Source: CAD feature listing. Evaluate the final solid. Frame: model axes, mm. A direction names the side the tool comes from. Round coordinates to 2 decimals unless told otherwise and drop trailing zeros. Write each loop counter-clockwise with the first axis right and the second up, starting at its lowest first coordinate (ties: lowest second). Pieces come first, ordered by that corner, then holes. Notation, with made-up numbers: (86, -24.5) - (95, -24.5) arc R16 ccw to (95, -16.5) - close; hole circle Ø2 at (89.25, 7). An arc over 180 degrees is marked (long way). Write item = value, one per line. Start each with the question number.
```python
from build123d import *

# Parameters (mm, degrees)
SKETCH1_W      = 16
SKETCH1_H      = 16
EXTRUDE1_DEPTH = 112
SKETCH2_W      = 13
SKETCH2_H      = 13
EXTRUDE2_DEPTH = 115.262854857
SKETCH3_R      = 4
SKETCH3_R_2    = 1.85
EXTRUDE3_DEPTH = 115.262854857
SKETCH4_R      = 4
SKETCH4_R_2    = 1.85
EXTRUDE4_DEPTH = 115.262854857
FILLET1_R      = 1


with BuildPart() as part:
    # Sketch1 → Extrude1 (new body)
    with BuildSketch(Plane.XY):
        with Locations((8, 8)):
            Rectangle(SKETCH1_W, SKETCH1_H)
    extrude(amount=-EXTRUDE1_DEPTH)

    # Sketch2 → Extrude2 (cut, through all)
    with BuildSketch(Plane.XY):
        with Locations((8, 8)):
            Rectangle(SKETCH2_W, SKETCH2_H)
    extrude(amount=-EXTRUDE2_DEPTH, mode=Mode.SUBTRACT)

    # Sketch3 → Extrude3 (cut, through all)
    with BuildSketch(Plane(origin=(0, 16, 0), x_dir=(1, 0, 0), z_dir=(0, 1, 0))):
        with Locations(Location((8, 64, 0), (0, 0, 270))):
            Circle(SKETCH3_R)
        with Locations(Location((8, 32, 0), (0, 0, 270))):
            Circle(SKETCH3_R)
        with Locations((8, 0)):
            Circle(SKETCH3_R)
        with Locations(Location((8, 96, 0), (0, 0, 270))):
            Circle(SKETCH3_R)
        with Locations((8, 128)):
            Circle(SKETCH3_R)
        with Locations((8, 160)):
            Circle(SKETCH3_R)
        with Locations((8, 192)):
            Circle(SKETCH3_R)
        with Locations((8, 224)):
            Circle(SKETCH3_R)
        with Locations((8, 256)):
            Circle(SKETCH3_R)
        with Locations(Location((8, 48, 0), (0, 0, 270))):
            Circle(SKETCH3_R)
        with Locations(Location((8, 56, 0), (0, 0, 270))):
            Circle(SKETCH3_R_2)
        with Locations(Location((8, 40, 0), (0, 0, 270))):
            Circle(SKETCH3_R_2)
        with Locations(Location((8, 80, 0), (0, 0, 270))):
            Circle(SKETCH3_R)
        with Locations(Location((8, 88, 0), (0, 0, 270))):
            Circle(SKETCH3_R_2)
        with Locations(Location((8, 72, 0), (0, 0, 270))):
            Circle(SKETCH3_R_2)
        with Locations(Location((8, 16, 0), (0, 0, 270))):
            Circle(SKETCH3_R)
        with Locations(Location((8, 24, 0), (0, 0, 270))):
            Circle(SKETCH3_R_2)
        with Locations(Location((8, 8, 0), (0, 0, 270))):
            Circle(SKETCH3_R_2)
        with Locations((8, 112)):
            Circle(SKETCH3_R)
        with Locations((8, 120)):
            Circle(SKETCH3_R_2)
        with Locations(Location((8, 104, 0), (0, 0, 270))):
            Circle(SKETCH3_R_2)
        with Locations((8, 144)):
            Circle(SKETCH3_R)
        with Locations((8, 152)):
            Circle(SKETCH3_R_2)
        with Locations((8, 136)):
            Circle(SKETCH3_R_2)
        with Locations((8, 176)):
            Circle(SKETCH3_R)
        with Locations((8, 184)):
            Circle(SKETCH3_R_2)
        with Locations((8, 168)):
            Circle(SKETCH3_R_2)
        with Locations((8, 208)):
            Circle(SKETCH3_R)
        with Locations((8, 216)):
            Circle(SKETCH3_R_2)
        with Locations((8, 200)):
            Circle(SKETCH3_R_2)
        with Locations((8, 240)):
            Circle(SKETCH3_R)
        with Locations((8, 248)):
            Circle(SKETCH3_R_2)
        with Locations((8, 232)):
            Circle(SKETCH3_R_2)
    extrude(amount=-EXTRUDE3_DEPTH, mode=Mode.SUBTRACT)

    # Sketch4 → Extrude4 (cut, through all)
    with BuildSketch(Plane(origin=(16, 0, 0), x_dir=(0, 0, -1), z_dir=(1, 0, 0))):
        with Locations(Location((32, 8, 0), (0, 0, 90))):
            Circle(SKETCH4_R)
        with Locations(Location((64, 8, 0), (0, 0, 90))):
            Circle(SKETCH4_R)
        with Locations((0, 8)):
            Circle(SKETCH4_R)
        with Locations(Location((96, 8, 0), (0, 0, 90))):
            Circle(SKETCH4_R)
        with Locations((128, 8)):
            Circle(SKETCH4_R)
        with Locations((160, 8)):
            Circle(SKETCH4_R)
        with Locations((192, 8)):
            Circle(SKETCH4_R)
        with Locations((224, 8)):
            Circle(SKETCH4_R)
        with Locations((256, 8)):
            Circle(SKETCH4_R)
        with Locations(Location((48, 8.074203, 0), (0, 0, 90))):
            Circle(SKETCH4_R)
        with Locations(Location((40, 8.074203, 0), (0, 0, 90))):
            Circle(SKETCH4_R_2)
        with Locations(Location((56, 8.074203, 0), (0, 0, 90))):
            Circle(SKETCH4_R_2)
        with Locations(Location((80, 8, 0), (0, 0, 90))):
            Circle(SKETCH4_R)
        with Locations(Location((72, 8, 0), (0, 0, 90))):
            Circle(SKETCH4_R_2)
        with Locations(Location((88, 8, 0), (0, 0, 90))):
            Circle(SKETCH4_R_2)
        with Locations(Location((16, 8, 0), (0, 0, 90))):
            Circle(SKETCH4_R)
        with Locations(Location((8, 8, 0), (0, 0, 90))):
            Circle(SKETCH4_R_2)
        with Locations(Location((24, 8, 0), (0, 0, 90))):
            Circle(SKETCH4_R_2)
        with Locations((112, 8)):
            Circle(SKETCH4_R)
        with Locations(Location((104, 8, 0), (0, 0, 90))):
            Circle(SKETCH4_R_2)
        with Locations((120, 8)):
            Circle(SKETCH4_R_2)
        with Locations((144, 8)):
            Circle(SKETCH4_R)
        with Locations((136, 8)):
            Circle(SKETCH4_R_2)
        with Locations((152, 8)):
            Circle(SKETCH4_R_2)
        with Locations((176, 8)):
            Circle(SKETCH4_R)
        with Locations((168, 8)):
            Circle(SKETCH4_R_2)
        with Locations((184, 8)):
            Circle(SKETCH4_R_2)
        with Locations((208, 8)):
            Circle(SKETCH4_R)
        with Locations((200, 8)):
            Circle(SKETCH4_R_2)
        with Locations((216, 8)):
            Circle(SKETCH4_R_2)
        with Locations((240, 8)):
            Circle(SKETCH4_R)
        with Locations((232, 8)):
            Circle(SKETCH4_R_2)
        with Locations((248, 8)):
            Circle(SKETCH4_R_2)
    extrude(amount=-EXTRUDE4_DEPTH, mode=Mode.SUBTRACT)

    # Fillet1
    fillet1_edges = [part.edges().sort_by_distance(p)[0] for p in [
        (0, 16, -56),
        (16, 16, -56),
        (16, 0, -56),
        (0, 0, -56),
    ]]
    fillet(fillet1_edges, radius=FILLET1_R)


solid = part.part
```
(1) Section D-D (y = 8.5). Count the separate pieces of the cut face and the enclosed holes in it, plus the area to 3 significant figures.
(2) Contact query for a flat-ended pin moving along its axis: P1, Ø4, axis at x = 13, y = 12, coming from the +Z side. Output: stop coordinate, or through.
(3) Section A-A (z = -48). Return the cut outline in (x, y), plus the area to 3 significant figures.
(4) Reachability of faces 1 (the flat face through (0, 6, -55)), 2 (the flat face through (5, 14.5, -55)) from +Z, -Z, +X, -X, +Y, -Y: full face, straight path, thin tool, end or side. Return the list, or none.
(5) Pull-direction query (Y, two-part tool) for faces 3 (the cylindrical face through (7.29, 15.26, -102.29)), 4 (the cylindrical face through (15.26, 7.479, -28.034)); classes: +Y half, -Y half, draft (parallel to the pull), parting line (faces both ways), or undercut.
(6) Ray query, L1, parallel to X at y = 3, z = -66.5; L2, parallel to X at y = 15, z = -35. Return the intervals inside material, ascending. Write a range as from..to.
(7) Section B-B (x = 3). Return the cut outline in (y, z), plus the area to 3 significant figures.
Solution:
q1.separate_pieces = 28
q1.enclosed_holes = 0
q1.area = 94.2 mm^2
q2.P1 = 0
q3.outline = (0, 1) arc R1 ccw to (1, 0) - (4, 0) - (4, 1.5) - (1.5, 1.5) - (1.5, 4.07) - (0, 4.07) - close; (0, 12.07) - (1.5, 12.07) - (1.5, 14.5) - (4, 14.5) - (4, 16) - (1, 16) arc R1 ccw to (0, 15) - close; (12, 0) - (15, 0) arc R1 ccw to (16, 1) - (16, 4.07) - (14.5, 4.07) - (14.5, 1.5) - (12, 1.5) - close; (12, 14.5) - (14.5, 14.5) - (14.5, 12.07) - (16, 12.07) - (16, 15) arc R1 ccw to (15, 16) - (12, 16) - close
q3.area = 38.1 mm^2
q4.face_1 = +Z, -Z, -X, +Y, -Y
q4.face_2 = +Z, -Z
q5.face_3 = draft
q5.face_4 = undercut
q6.L1 = 0..1.5, 14.5..16
q6.L2 = 0..5.35, 10.65..16
q7.outline = (0, -112) - (1.5, -112) - (1.5, 0) - (0, 0) - close; (14.5, -112) - (16, -112) - (16, 0) - (14.5, 0) - close
q7.area = 336 mm^2
